For this review, take the finished solid that the model builds, in its own axes (mm). A direction names the side the tool comes from. Give positions to 0.01 mm unless a question says otherwise; leave off trailing zeros. Order: outer loops, then holes, each group sorted by start corner. A loop starts at its lowest first (then second) coordinate and runs counter-clockwise, first axis right, second up. Notation, with made-up numbers: M -12,-23.75 L 0,-23.75 A20 ccw 0,-19.75 Z; hole C -13.5,86 d5. An arc over 180 degrees is marked long. Use CSV: the item, a comma, the result in double quotes. Start each with the question number.
(1) Consider section D-D (y = 15.5). Write out the cut boundary in (x, z), and give its area (3 significant figures).
(2) Tool access review of faces 4 (the face through (30, 45, 90)), 5 (the face through (30, 27, 55)), 6 (the face through (30, -10, 32)): name each direction out of +Z, -Z, +X, -X, +Y, -Y from which nothing blocks a thin tool from reaching the whole face with its end or side.
(3) Clearance check with flat-ended pins moving along their axes: P1, Ø6, axis at x = 30.5, y = 19.5, coming from the -Z side; P2, Ø10, axis at x = 55, y = -16.5, coming from the +Z side; P3, Ø10, axis at x = 31, z = 85.5, coming from the -Y side; P4, Ø10, axis at x = 23.5, y = -18.5, coming from the +Z side. State where each tip first meets the part, or that it passes through.
(4) Consider section B-B (x = 33). Write out the cut boundary in (y, z), and give its area (3 significant figures).
(5) Draft analysis for pull direction X (two halves, no side actions). For faces 1 (the face through (20, 34, 63)), 2 (the face through (50, -30, 5)), 3 (the face through (6, -19, 10)), state which applies: pulls with the +X half, pulls with the -X half, needs draft (parallel to the pull), parting line crosses it, or undercut.
(6) Consider section C-C (z = 107.5). Write out the cut boundary in (x, y), and give its area (3 significant figures).
(7) Consider section A-A (y = -13). Write out the cut boundary in (x, z).
(8) Wall thickness on L1, parallel to Y at x = 29, z = 107; L2, parallel to X at y = -20, z = 8; L3, parallel to Z at x = 3.5, y = -2: over which ranges is each line inside the solid? List them lowest first. Write a range as from..to.
```python
from build123d import *

# Parameters (mm, degrees)
P_IDAT_VYSUNUT_M1_DEPTH  = 10
SKICA2_W                 = 20
SKICA2_H                 = 10
P_IDAT_VYSUNUT_M2_DEPTH  = 55
SKICA4_W                 = 20
SKICA4_H                 = 10
P_IDAT_VYSUNUT_M3_DEPTH  = 55
SKICA5_W                 = 20
SKICA5_H                 = 10
P_IDAT_VYSUNUT_M4_DEPTH  = 50
SKICA6_W                 = 20
SKICA6_H                 = 15
P_IDAT_VYSUNUT_M5_DEPTH  = 30
SKICA7_R                 = 5
ODEBRAT_VYSUNUT_M1_DEPTH = 20


with BuildPart() as part:
    # Skica1 → Přidat vysunutím1 (new body)
    with BuildSketch(Plane.XY):
        Polygon((0, 0), (60, 0), (60, -50), (50, -50), (50, -10), (10, -10), (10, -50), (0, -50), align=None)
    extrude(amount=P_IDAT_VYSUNUT_M1_DEPTH)

    # Skica2 → Přidat vysunutím2 (add)
    with BuildSketch(Plane.XY.offset(10)):
        with Locations((30, -5)):
            Rectangle(SKICA2_W, SKICA2_H)
    extrude(amount=P_IDAT_VYSUNUT_M2_DEPTH)

    # Skica4 → Přidat vysunutím3 (add)
    with BuildSketch(Plane(origin=(0, 0, 0), x_dir=(1, 0, 0), z_dir=(0, 1, 0))):
        with Locations((30, -60)):
            Rectangle(SKICA4_W, SKICA4_H)
    extrude(amount=P_IDAT_VYSUNUT_M3_DEPTH)

    # Skica5 → Přidat vysunutím4 (add)
    with BuildSketch(Plane.XY.offset(65)):
        with Locations((30, 50)):
            Rectangle(SKICA5_W, SKICA5_H)
    extrude(amount=P_IDAT_VYSUNUT_M4_DEPTH)

    # Skica6 → Přidat vysunutím5 (add)
    with BuildSketch(Plane(origin=(0, 55, 0), x_dir=(1, 0, 0), z_dir=(0, 1, 0))):
        with Locations((30, -107.5)):
            Rectangle(SKICA6_W, SKICA6_H)
    extrude(amount=P_IDAT_VYSUNUT_M5_DEPTH)

    # Skica7 → Odebrat vysunutím1 (cut)
    with BuildSketch(Plane(origin=(40, 0, 0), x_dir=(0, 0, -1), z_dir=(1, 0, 0))):
        with Locations((-107.5, 77)):
            Circle(SKICA7_R)
    extrude(amount=-ODEBRAT_VYSUNUT_M1_DEPTH, mode=Mode.SUBTRACT)


solid = part.part
```
Check result:
1,outline,"M 20,55 L 40,55 L 40,65 L 20,65 Z"
1,area,"200 mm^2"
2,face 4,"+Z, +X, -X, -Y"
2,face 5,"-Z, +X, -X, +Y"
2,face 6,"+Z, -Z, -Y"
3,P1,"stops at z = 55"
3,P2,"stops at z = 10"
3,P3,"stops at y = 45"
3,P4,"passes through"
4,outline,"M -10,0 L 0,0 L 0,55 L 55,55 L 55,100 L 85,100 L 85,115 L 45,115 L 45,65 L -10,65 Z; hole C 77,107.5 d10"
4,area,"2,070 mm^2"
5,face 1,"pulls with the -X half"
5,face 2,"undercut"
5,face 3,"needs draft"
6,outline,"M 20,45 L 40,45 L 40,72 L 20,72 Z; M 20,82 L 40,82 L 40,85 L 20,85 Z"
6,area,"600 mm^2"
7,outline,"M 0,0 L 10,0 L 10,10 L 0,10 Z; M 50,0 L 60,0 L 60,10 L 50,10 Z"
8,L1,"y = 45..72.03, 81.97..85"
8,L2,"x = 0..10, 50..60"
8,L3,"z = 0..10"
